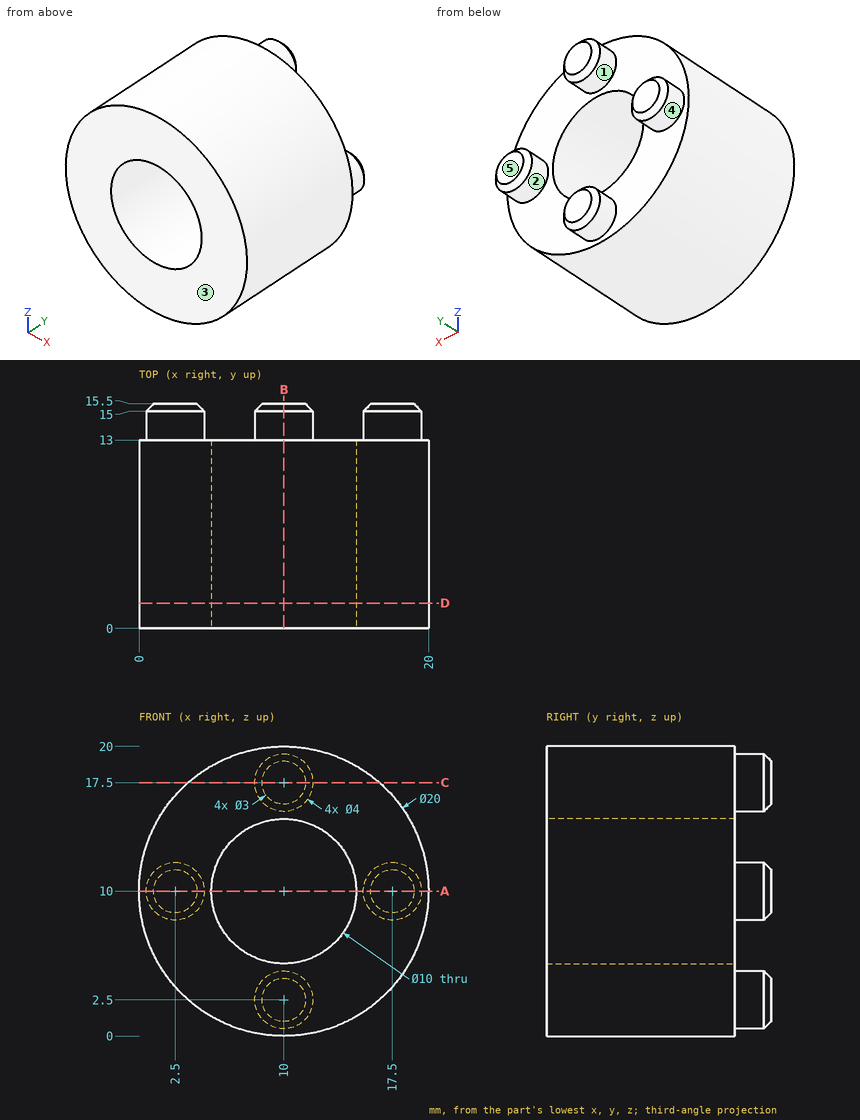
For this review, use the dimensioned drawing (mm, ordinates from the lowest corner) and the shaded views. A direction names the side the tool comes from. Coordinates: 2 decimals unless noted, no trailing zeros. Loops run counter-clockwise (first coordinate to the right, second up) from the corner with the lowest first, then second, coordinate; pieces in that order, holes last.
1. Add section B-B, the plane x = 10. Give the boundary of the cut face in (y, z).
2. For the marked faces 4 and 5, list the 3-axis set-ups (+Z, -Z, +X, -X, +Y, -Y) from which the entire face can be reached by the end or side of a thin tool; tool diameter is ignored.
3. Add section C-C, the plane z = 17.5. Give the boundary of the cut face in (x, y).
4. Add section A-A, the plane z = 10. Give the boundary of the cut face in (x, y), then the cut area to 4 significant figures.
5. For line 1 (Z direction, x = 9.75, y = 4.5); line 2 (X direction, y = 3, z = 10); line 3 (X direction, y = 9.75, z = 8.75), list the stretches that pass through material, from the lowest coordinate up.
6. Insertion check: P1, Ø8, axis at x = 17.5, z = 16.5, coming from the -Y side; P2, Ø2, axis at y = 13.5, z = 8, coming from the -X side; P3, Ø3, axis at y = 3, z = 5, coming from the +X side; P4, Ø6, axis at x = 9, z = 12.5, coming from the +Y side. Each pin has a flat end and moves straight along its axis. Give the tip position at first contact, or say it passes through.
7. Add section D-D, the plane y = 1.75. Give the boundary of the cut face in (x, z).
8. Mouldability with a two-part tool opening along X and no side actions: class the marked faces 1, 2 and 3 as +X half, -X half, draft (parallel to the pull), parting line (faces both ways), or undercut.
Result:
1. outline: (0, 0) - (13, 0) - (13, 0.5) - (15, 0.5) - (15.5, 1) - (15.5, 4) - (15, 4.5) - (13, 4.5) - (13, 5) - (0, 5) - close; (0, 15) - (13, 15) - (13, 15.5) - (15, 15.5) - (15.5, 16) - (15.5, 19) - (15, 19.5) - (13, 19.5) - (13, 20) - (0, 20) - close
2. face 4: +Y
2. face 5: +Z, -Z, +X, -X, +Y
3. outline: (3.39, 0) - (16.61, 0) - (16.61, 13) - (12, 13) - (12, 15) - (11.5, 15.5) - (8.5, 15.5) - (8, 15) - (8, 13) - (3.39, 13) - close
4. outline: (0, 0) - (5, 0) - (5, 13) - (4.5, 13) - (4.5, 15) - (4, 15.5) - (1, 15.5) - (0.5, 15) - (0.5, 13) - (0, 13) - close; (15, 0) - (20, 0) - (20, 13) - (19.5, 13) - (19.5, 15) - (19, 15.5) - (16, 15.5) - (15.5, 15) - (15.5, 13) - (15, 13) - close
4. area: 149.5 mm2
5. line 1: z = 0 to 5.01, 14.99 to 20
5. line 2: x = 0 to 5, 15 to 20
5. line 3: x = 0.08 to 5.16, 14.84 to 19.92
6. P1: stops at y = 0
6. P2: stops at x = 0.06
6. P3: stops at x = 19.37
6. P4: stops at y = 13
7. outline: circle Ø20 at (10, 10); hole circle Ø10 at (10, 10)
8. face 1: parting line
8. face 2: undercut
8. face 3: draft
